```python
from build123d import *

# Parameters (mm, degrees)
SKETCH_W                   = 74
SKETCH_H                   = 74
PAD_DEPTH                  = 3
SKETCH002_W                = 64
SKETCH002_H                = 64
SKETCH002_W_2              = 60
SKETCH002_H_2              = 60
PAD001_DEPTH               = 35
SKETCH003_R                = 1.5
POCKET_DEPTH               = 225.675651
PAD002_DEPTH               = 32
SKETCH005_R                = 2.4
POCKET001_DEPTH            = 10
SKETCH003_MIRRORED_2_R     = 1.5
POCKET_MIRRORED_2_DEPTH    = 225.675651
PAD002_MIRRORED_2_DEPTH    = 32
SKETCH005_MIRRORED_2_R     = 2.4
POCKET001_MIRRORED_2_DEPTH = 10
SKETCH006_R                = 3.25
POCKET002_DEPTH            = 38.001
SKETCH008_R                = 4
POCKET003_DEPTH            = 2.5
SKETCH009_R                = 6
PAD003_DEPTH               = 3
SKETCH010_R                = 3.25
POCKET004_DEPTH            = 6.001
SKETCH011_R                = 3.25
POCKET005_DEPTH            = 38.001
SKETCH012_W                = 8
SKETCH012_H                = 6
POCKET006_DEPTH            = 1
SKETCH013_W                = 5
SKETCH013_H                = 5
PAD004_DEPTH               = 16


with BuildPart() as part:
    # Sketch → Pad (new body)
    with BuildSketch(Plane.XY):
        Rectangle(SKETCH_W, SKETCH_H)
    extrude(amount=PAD_DEPTH)

    # Sketch002 (on Face5 of Pad) → Pad001 (join)
    with BuildSketch(Plane(origin=(0, 0, 0), x_dir=(1, 0, 0), z_dir=(0, 0, -1))):
        Rectangle(SKETCH002_W, SKETCH002_H)
        Rectangle(SKETCH002_W_2, SKETCH002_H_2, mode=Mode.SUBTRACT)
    extrude(amount=PAD001_DEPTH)

    # Sketch003 (on Face4 of Pad001) → Pocket (cut, through all)
    with BuildSketch(Plane(origin=(0, 0, 0), x_dir=(1, 0, 0), z_dir=(0, 0, -1))):
        with Locations((-34, 34)):
            Circle(SKETCH003_R)
    pocket = extrude(amount=-POCKET_DEPTH, mode=Mode.SUBTRACT)

    # Sketch004 (on Face17 of Pocket) → Pad002 (join)
    with BuildSketch(Plane(origin=(0, 0, 0), x_dir=(1, 0, 0), z_dir=(0, 0, -1))):
        with BuildLine():
            ThreePointArc((-30, 22), (-24.343146, 24.343146), (-22, 30))
            Line((-30, 30), (-22, 30))
            Line((-30, 30), (-30, 22))
        make_face()
    pad002 = extrude(amount=PAD002_DEPTH)

    # Sketch005 (on Face17 of Pad002) → Pocket001 (cut)
    with BuildSketch(Plane(origin=(0, 0, -32), x_dir=(1, 0, 0), z_dir=(0, 0, -1))):
        with Locations((-27, 27)):
            Circle(SKETCH005_R)
    pocket001 = extrude(amount=-POCKET001_DEPTH, mode=Mode.SUBTRACT)

    # Sketch003 Mirrored 2 → Pocket Mirrored 2 (cut, through all)
    with BuildSketch(Plane(origin=(0, 0, 0), x_dir=(-1, 0, 0), z_dir=(0, 0, 1))):
        with Locations((-34, 34)):
            Circle(SKETCH003_MIRRORED_2_R)
    pocket_mirrored_2 = extrude(amount=POCKET_MIRRORED_2_DEPTH, mode=Mode.SUBTRACT)

    # Sketch004 Mirrored 2 → Pad002 Mirrored 2 (add)
    with BuildSketch(Plane(origin=(0, 0, 0), x_dir=(-1, 0, 0), z_dir=(0, 0, 1))):
        with BuildLine():
            ThreePointArc((-30, 22), (-24.343146, 24.343146), (-22, 30))
            Line((-30, 30), (-22, 30))
            Line((-30, 30), (-30, 22))
        make_face()
    pad002_mirrored_2 = extrude(amount=-PAD002_MIRRORED_2_DEPTH)

    # Sketch005 Mirrored 2 → Pocket001 Mirrored 2 (cut)
    with BuildSketch(Plane(origin=(0, 0, -32), x_dir=(-1, 0, 0), z_dir=(0, 0, 1))):
        with Locations((-27, 27)):
            Circle(SKETCH005_MIRRORED_2_R)
    pocket001_mirrored_2 = extrude(amount=POCKET001_MIRRORED_2_DEPTH, mode=Mode.SUBTRACT)

    # Mirrored001: Pocket, Pad002, Pocket001, Pocket Mirrored 2, Pad002 Mirrored 2, Pocket001 Mirrored 2 across Sketch003 H_Axis
    add(pocket.mirror(Plane(origin=(0, 0, 0), x_dir=(0, 0, -1), z_dir=(0, -1, 0))), mode=Mode.SUBTRACT)
    add(pad002.mirror(Plane(origin=(0, 0, 0), x_dir=(0, 0, -1), z_dir=(0, -1, 0))))
    add(pocket001.mirror(Plane(origin=(0, 0, 0), x_dir=(0, 0, -1), z_dir=(0, -1, 0))), mode=Mode.SUBTRACT)
    add(pocket_mirrored_2.mirror(Plane(origin=(0, 0, 0), x_dir=(0, 0, -1), z_dir=(0, -1, 0))), mode=Mode.SUBTRACT)
    add(pad002_mirrored_2.mirror(Plane(origin=(0, 0, 0), x_dir=(0, 0, -1), z_dir=(0, -1, 0))))
    add(pocket001_mirrored_2.mirror(Plane(origin=(0, 0, 0), x_dir=(0, 0, -1), z_dir=(0, -1, 0))), mode=Mode.SUBTRACT)

    # Sketch006 (on Face36 of MultiTransform) → Pocket002 (cut, through all)
    with BuildSketch(Plane.XY.offset(3)):
        with Locations((0, -1)):
            Circle(SKETCH006_R)
    extrude(amount=-POCKET002_DEPTH, mode=Mode.SUBTRACT)

    # Sketch008 (on Face23 of Pocket002) → Pocket003 (cut)
    with BuildSketch(Plane.XY.offset(3)):
        with Locations((-18.5, -7)):
            Circle(SKETCH008_R)
        with Locations((18.5, -7)):
            Circle(SKETCH008_R)
    extrude(amount=-POCKET003_DEPTH, mode=Mode.SUBTRACT)

    # Sketch009 (on Face4 of Pocket003) → Pad003 (join)
    with BuildSketch(Plane(origin=(0, 0, 0), x_dir=(1, 0, 0), z_dir=(0, 0, -1))):
        with Locations((18.5, 7)):
            Circle(SKETCH009_R)
        with Locations((-18.5, 7)):
            Circle(SKETCH009_R)
    extrude(amount=PAD003_DEPTH)

    # Sketch010 (on Face25 of Pad003) → Pocket004 (cut, through all)
    with BuildSketch(Plane(origin=(0, 0, -3), x_dir=(1, 0, 0), z_dir=(0, 0, -1))):
        with Locations((-18.5, 7)):
            Circle(SKETCH010_R)
    extrude(amount=-POCKET004_DEPTH, mode=Mode.SUBTRACT)

    # Sketch011 (on Face27 of Pocket004) → Pocket005 (cut, through all)
    with BuildSketch(Plane.XY.offset(3)):
        with Locations((18.5, -7)):
            Circle(SKETCH011_R)
    extrude(amount=-POCKET005_DEPTH, mode=Mode.SUBTRACT)

    # Sketch012 (on Face27 of Pocket005) → Pocket006 (cut)
    with BuildSketch(Plane.XY.offset(3)):
        with Locations((-18.5, 6)):
            Rectangle(SKETCH012_W, SKETCH012_H)
        Polygon((-22.6, 1), (-22.6, 11), (-31.260254, 6), align=None)
    pocket006 = extrude(amount=-POCKET006_DEPTH, mode=Mode.SUBTRACT)

    # Mirrored002: Pocket006 across Sketch012 V_Axis
    add(pocket006.mirror(Plane(origin=(0, 0, 3), x_dir=(0, 0, 1), z_dir=(1, 0, 0))), mode=Mode.SUBTRACT)

    # Sketch013 (on Face4 of MultiTransform001) → Pad004 (join)
    with BuildSketch(Plane(origin=(0, 0, 0), x_dir=(1, 0, 0), z_dir=(0, 0, -1))):
        with Locations((-27.5, -19.5)):
            Rectangle(SKETCH013_W, SKETCH013_H)
        with Locations((17.5, -2.5)):
            Rectangle(SKETCH013_W, SKETCH013_H)
    extrude(amount=PAD004_DEPTH)


solid = part.part
```
Model file for the job. Use its own axes, mm. A direction names the side the tool comes from. Coordinates: 2 decimals unless noted, no trailing zeros. Order: outer loops, then holes, each group sorted by start corner. A loop starts at its lowest first (then second) coordinate and runs counter-clockwise, first axis right, second up. Notation, with made-up numbers: (70, 77.25) - (76, 77.25) arc R23 cw to (76, 96.25) - close; hole circle Ø1 at (50, 50). An arc over 180 degrees is marked (long way). Return JSON: item names as keys, results as strings. Group by question number.
1) Probe line 1 (X direction, y = 34, z = 2.2); line 2 (X direction, y = 1, z = -9). List the from-to ranges inside material, lowest first. Write a range as from..to.
2) Flat gauge pins, fed straight in: P1, Ø8, axis at y = 5, z = -5.5, coming from the +X side; P2, Ø2.5, axis at y = 2.5, z = -11, coming from the -X side; P3, Ø12, axis at x = -17, y = 11.5, coming from the -Z side. Where does each tip first touch, or does it go through?
3) Mould opens along X. For faces 1 (the flat face through (26, 6, 2)), 2 (the flat face through (-3, 31, -35)) say: released by +X, released by -X, zero draft, split by the parting line, or undercut.
4) Saw through at C-C, the plane y = -16. Write the cut outline in (x, z), plus the area to 3 significant figures.
5) Tool access for faces 3 (the cylindrical face through (-21.747, -7.143, -1.274)), 4 (the flat face through (0, -32, -17)), 5 (the flat face through (22, -7, 0.5)), 6 (the flat face through (-1, -37, 1)), 7 (the flat face through (0, 7, 0)): list every direction of +Z, -Z, +X, -X, +Y, -Y with a clear straight run to the whole face (end or side of a thin tool).
6) Saw through at A-A, the plane y = 34. Write the cut outline in (x, z), plus the area to 3 significant figures.
Values found:
{
 "1": {"line 1": "x = -37..-35.5, -32.5..32.5, 35.5..37", "line 2": "x = -32..-30, 15..20, 30..32"},
 "2": {"P1": "stops at x = 32", "P2": "stops at x = -32", "P3": "stops at z = 0"},
 "3": {"face 1": "undercut", "face 2": "zero draft"},
 "4": {"outline": "(-37, 0) - (-32, 0) - (-32, -35) - (-30, -35) - (-30, 0) - (30, 0) - (30, -35) - (32, -35) - (32, 0) - (37, 0) - (37, 3) - (-37, 3) - close", "area": "362 mm²"},
 "5": {"face 3": "+Z, -Z", "face 4": "-Z, +X, -X, -Y", "face 5": "+Z", "face 6": "+Z, -Z, +X, -X, -Y", "face 7": "-Z"},
 "6": {"outline": "(-37, 0) - (-35.5, 0) - (-35.5, 3) - (-37, 3) - close; (-32.5, 0) - (32.5, 0) - (32.5, 3) - (-32.5, 3) - close; (35.5, 0) - (37, 0) - (37, 3) - (35.5, 3) - close", "area": "204 mm²"}
}
